```python
from build123d import *

# Parameters (mm, degrees)
CUT_EXTRUDE1_DEPTH = 5.7
CIRPATTERN1_COUNT  = 15


with BuildPart() as part:
    # Sketch1 → 52 Tooth (revolve)
    with BuildSketch(Plane.XY, mode=Mode.PRIVATE) as f_52_tooth_sk:
        Polygon((12.827, 0), (12.827, 10), (11, 10), (11, 8), (5.375, 8), (5.375, 16.4), (4, 16.4), (4, 21.8), (3.85, 21.8), (3.85, 27.5), (0, 27.5), (0, 14.75), (3.55, 14.75), (3.55, 3.5), (7, 3.5), (7, 0), align=None)
    revolve(f_52_tooth_sk.sketch.rotate(Axis((0, 0, 0), (0, 1, 0)), 90), axis=Axis((0, 0, 0), (0, 1, 0)))

    # Sketch2 → Cut-Extrude1 (cut)
    with BuildSketch(Plane(origin=(0, 27.5, 0), x_dir=(1, 0, 0), z_dir=(0, 1, 0))):
        with BuildLine():
            ThreePointArc((0.80046001, 3.765868263), (0, 3.85), (-0.80046001, 3.765868263))
            Line((-0.80046001, 3.765868263), (0, 3.25))
            Line((0, 3.25), (0.80046001, 3.765868263))
        make_face()
    cut_extrude1 = extrude(amount=-CUT_EXTRUDE1_DEPTH, mode=Mode.SUBTRACT)

    # CirPattern1: Cut-Extrude1 ×15 about axis
    cirpattern1_axis = Axis((0, 0, 0), (0, 1, 0))
    for i in range(1, CIRPATTERN1_COUNT):
        add(cut_extrude1.rotate(cirpattern1_axis, i * 360 / CIRPATTERN1_COUNT), mode=Mode.SUBTRACT)


solid = part.part
```
The model under review builds one solid part; all positions refer to its coordinate system, in mm. A direction names the side the tool comes from. Round coordinates to 2 decimals unless told otherwise and drop trailing zeros. Write each loop counter-clockwise with the first axis right and the second up, starting at its lowest first coordinate (ties: lowest second). Pieces come first, ordered by that corner, then holes. Notation, with made-up numbers: M 5.25,-32.5 L 25.25,-32.5 A21 cw 25.25,-13.5 Z; hole C 55.25,12 d6. An arc over 180 degrees is marked long. Use CSV: the item, a comma, the result in double quotes. Start each with the question number.
(1) Clearance check with flat-ended pins moving along their axes: P1, Ø8, axis at y = 8, z = -1.5, coming from the -X side; P2, Ø12, axis at y = 13, z = -9, coming from the +X side; P3, Ø3, axis at x = 2, y = 13, coming from the -Z side; P4, Ø5.5, axis at x = 0.5, z = -0.5, coming from the -Y side. State where each tip first meets the part, or that it passes through.
(2) Tool access review of faces 4 (the face through (0.39, 24.69, -3.5)), 5 (the face through (-2.84, 24.69, 2.11)), 6 (the face through (-10, 10, -6)), 7 (the face through (3, 3.5, 3)): name each direction out of +Z, -Z, +X, -X, +Y, -Y from which nothing blocks a thin tool from reaching the whole face with its end or side.
(3) The part is to be moulded in two halves that separate along Z. For faces 1 (the face through (3.444, 24.69, 0.759)), 2 (the face through (2, 16.4, 4)), 3 (the face through (-2.88, 24.69, -2.05)), say which applies: +Z half, -Z half, draft (parallel to the pull), parting line (faces both ways), or undercut.
(4) For line 1 along X through (y, z) = (9.2, 0) (3 decimals); line 2 along X through (y, z) = (12.5, 0) (3 decimals); line 3 along X through (y, z) = (6.5, 0), list the stretches that pass through material, from the lowest coordinate up.
(5) We need section C-C, the plane y = 17. State the section outline as (x, z) points, then the cut area to 3 significant figures.
(6) We need section D-D, the plane y = 5. State the section outline as (x, z) points, then the cut area to 3 significant figures.
(7) We need section A-A, the plane y = 2.25. State the section outline as (x, z) points, then the cut area to 3 significant figures.
(8) We need section B-B, the plane z = -6.5. State the section outline as (x, y) points, then the cut area to 3 significant figures.
Findings:
1,P1,"x = -12.83"
1,P2,"x = 12.25"
1,P3,"z = -5.35"
1,P4,"y = 14.75"
2,face 4,"-Z, +Y"
2,face 5,"-X, +Y"
2,face 6,"+Y"
2,face 7,"-Y"
3,face 1,"undercut"
3,face 2,"draft"
3,face 3,"-Z half"
4,line 1,"-12.827 to -11, -5.375 to -3.55, 3.55 to 5.375, 11 to 12.827"
4,line 2,"-5.375 to -3.55, 3.55 to 5.375"
4,line 3,"-12.83 to -3.55, 3.55 to 12.83"
5,outline,"C 0,0 d8"
5,area,"50.3 mm^2"
6,outline,"C 0,0 d25.65; hole C 0,0 d7.1"
6,area,"477 mm^2"
7,outline,"C 0,0 d25.65; hole C 0,0 d14"
7,area,"363 mm^2"
8,outline,"M -11.06,0 L -2.6,0 L -2.6,3.5 L 2.6,3.5 L 2.6,0 L 11.06,0 L 11.06,10 L 8.87,10 L 8.87,8 L -8.87,8 L -8.87,10 L -11.06,10 Z"
8,area,"167 mm^2"
